Could you check a few things on this model? Use its own coordinates, in mm. A direction names the side the tool comes from. Coordinates: 2 decimals unless noted, no trailing zeros. Order: outer loops, then holes, each group sorted by start corner. A loop starts at its lowest first (then second) coordinate and runs counter-clockwise, first axis right, second up. Notation, with made-up numbers: M 5,10 L 62,10 A26 ccw 62,33 Z; hole C 2,14.25 d9. An arc over 180 degrees is marked long. Write item = value, one per line. Start each with the question number.
from build123d import *

# Parameters (mm, degrees)
BOSS_EXTRUDE2_DEPTH = 11
SKETCH4_R           = 1.5
CUT_EXTRUDE1_DEPTH  = 11


with BuildPart() as part:
    # Sketch1 → Boss-Extrude2 (new body)
    with BuildSketch(Plane.XY):
        Polygon((0, 0), (-20, 0), (-20, 60), (-17, 60), (-5, 60), (-5, 57), (-17, 57), (-17, 53.232919745), (-8, 53.232919745), (-8, 55.232919745), (-5, 55.232919745), (-5, 50.232919745), (-17, 50.232919745), (-17, 46.232919745), (-8, 46.232919745), (-8, 48.232919745), (-5, 48.232919745), (-5, 43.232919745), (-17, 43.232919745), (-17, 39.232919745), (-8, 39.232919745), (-8, 41.232919745), (-5, 41.232919745), (-5, 36.232919745), (-17, 36.232919745), (-17, 32.232919745), (-8, 32.232919745), (-8, 34.232919745), (-5, 34.232919745), (-5, 29.232919745), (-17, 29.232919745), (-17, 25.232919745), (-8, 25.232919745), (-8, 27.232919745), (-5, 27.232919745), (-5, 22.232919745), (-17, 22.232919745), (-17, 18.232919745), (-8, 18.232919745), (-8, 20.232919745), (-5, 20.232919745), (-5, 15.232919745), (-17, 15.232919745), (-17, 3), (0, 3), align=None)
    extrude(amount=BOSS_EXTRUDE2_DEPTH)

    # Sketch4 → Cut-Extrude1 (cut)
    with BuildSketch(Plane.XZ):
        with Locations((-3.103292827, 5.5)):
            Circle(SKETCH4_R)
        with Locations((-13.103292827, 5.5)):
            Circle(SKETCH4_R)
    extrude(amount=-CUT_EXTRUDE1_DEPTH, mode=Mode.SUBTRACT)


solid = part.part
(1) Imagine slicing it at A-A on x = -6.5. Give the number of separate pieces and of enclosed holes in the cut face, plus the area to 3 significant figures.
(2) Please list where these lines run through material, in increasing order: probe 1 along X at (y, z) = (48, 6.5); probe 2 along X at (y, z) = (49, 9.5); probe 3 along Y at (x, z) = (-2, 3). Write a range as from..to.
(3) For faces 1 (the flat face through (-11, 29.233, 5)), 2 (the flat face through (0, 2, 5)), 3 (the flat face through (-13, 53.233, 5)), which set-ups out of +Z, -Z, +X, -X, +Y, -Y let a thin tool reach every point of the face, with its end or its side?
(4) Imagine slicing it at B-B on x = -3. List the corners of the cut face in (y, z) for me.
(5) Thinking about a two-plate mould opening in Y: for faces 4 (the flat face through (-12, 60, 5)), 5 (the flat face through (-8, 40, 5)), 6 (the flat face through (-5, 25, 5)), 7 (the flat face through (-13, 46.233, 5)), which applies, released by +Y, released by -Y, zero draft, split by the parting line, or undercut?
(6) Will these pins go through, and if not, where does the flat tip stop? P1, Ø2.5, axis at y = 25, z = 3.5, coming from the +X side; P2, Ø2, axis at x = -10, y = 18, coming from the -Z side.
Response:
q1.separate_pieces = 8
q1.enclosed_holes = 0
q1.area = 396 mm2
q2.probe_1 = -20..-17, -8..-5
q2.probe_2 = -20..-17
q2.probe_3 = 0..3
q3.face_1 = +Z, -Z, +X
q3.face_2 = +Z, -Z, +X, +Y, -Y
q3.face_3 = +Z, -Z
q4.outline = M 0,0 L 3,0 L 3,4 L 0,4 Z; M 0,7 L 3,7 L 3,11 L 0,11 Z
q5.face_4 = released by +Y
q5.face_5 = undercut
q5.face_6 = zero draft
q5.face_7 = undercut
q6.P1 = -5
q6.P2 = 0
